Job drawing, mm, ordinate dimensions from the low corner. One solid piece. A direction names the side the tool comes from. Round coordinates to 2 decimals unless told otherwise and drop trailing zeros. Write each loop counter-clockwise with the first axis right and the second up, starting at its lowest first coordinate (ties: lowest second). Pieces come first, ordered by that corner, then holes. Notation, with made-up numbers: (84, 2.25) -> (131, 2.25) arc R20 ccw to (131, 13.25) -> close; hole circle Ø5 at (36.25, 37). An arc over 180 degrees is marked (long way). Use CSV: the item, a comma, the result in double quotes. Start each with the question number.
(1) Probe line 1 (Z direction, x = 1.3, y = 7.62); line 2 (X direction, y = 13.25, z = 7.25); line 3 (Z direction, x = 6.75, y = 8.5). List the from-to ranges inside material, lowest first. Write a range as [from, to].
(2) Drop flat-ended pins along their axis: pin 1 (5 mm diameter, centred on y = 8, z = 8.5, fed in from +X); pin 2 (5 mm diameter, centred on y = 2, z = 8, fed in from -X); pin 3 (3 mm diameter, centred on x = 13.5, y = 6, fed in from -Z); pin 4 (5 mm diameter, centred on x = 6, y = 2, fed in from -Z). Give the stop position or say it passes through.
(3) Which spindle directions (+Z, -Z, +X, -X, +Y, -Y) get a long thin tool onto all of the face, cutting with end or side? Do the marked faces 4, 5 and 6. Say none if no direction does.
(4) Saw through at C-C (x = 15.38). Give the cut face in (y, z).
(5) Saw through at B-B (z = 5.5). Give the cut face in (x, y) (1 decimal).
(6) Two-plate mould, pull along Y, no slides. Class the marked faces 1, 2 and 3: released by +Y, released by -Y, zero draft, split by the parting line, or undercut.
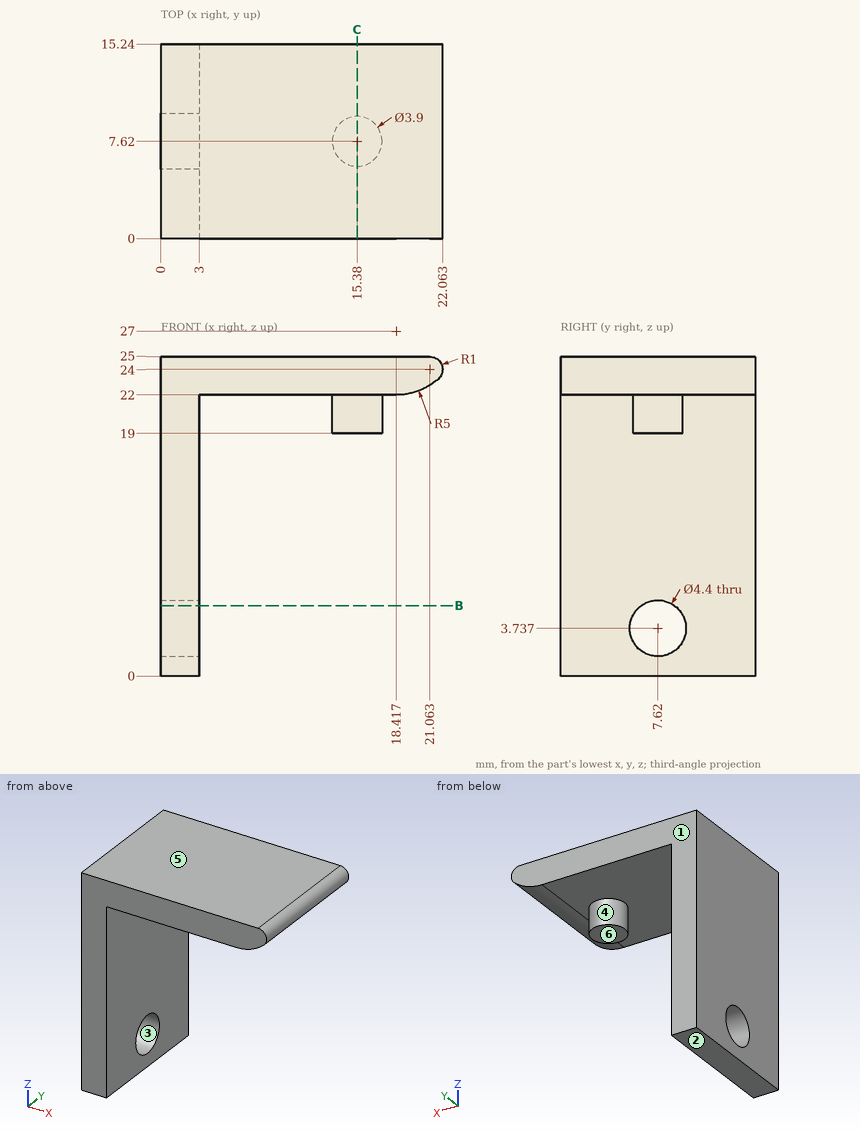
Answers:
1,line 1,"z = [0, 1.54], [5.94, 25]"
1,line 2,"x = [0, 3]"
1,line 3,"z = [22, 25]"
2,pin 1,"stops at x = 3"
2,pin 2,"stops at x = 0"
2,pin 3,"stops at z = 19"
2,pin 4,"stops at z = 22"
3,face 4,"-Z"
3,face 5,"+Z, +X, -X, +Y, -Y"
3,face 6,"-Z, +X, +Y, -Y"
4,outline,"(0, 22) -> (5.67, 22) -> (5.67, 19) -> (9.57, 19) -> (9.57, 22) -> (15.24, 22) -> (15.24, 25) -> (0, 25) -> close"
5,outline,"(0, 0) -> (3, 0) -> (3, 6.3) -> (0, 6.3) -> close; (0, 8.9) -> (3, 8.9) -> (3, 15.2) -> (0, 15.2) -> close"
6,face 1,"released by +Y"
6,face 2,"zero draft"
6,face 3,"undercut"
